Here's how the part is built. I have some questions about the finished solid (model axes, mm). Coordinates: 2 decimals unless noted, no trailing zeros. Order: outer loops, then holes, each group sorted by start corner. A loop starts at its lowest first (then second) coordinate and runs counter-clockwise, first axis right, second up. Notation, with made-up numbers: (29.5, 0.25) - (85.5, 0.25) arc R14 cw to (85.5, 6.25) - close; hole circle Ø10 at (2.5, 27). An arc over 180 degrees is marked (long way). Answer as CSV lines item,"result". Start each with the question number.
Q1. For pin 1 Ø1 at (y, z) = (-3, 29.5) entering from +X; pin 2 Ø1.5 at (x, z) = (-2.5, 28) entering from -Y, each with a flat end and sliding along its axis, tell me the tip position at first contact or that it passes through.
Q2. Suppose I cut it at B-B (z = 29.5). Please give me the cut outline in (x, y).
Q3. Thinking about a two-plate mould opening in Y: for faces 1 (the face through (6.466, -2.681, 28.779)), 2 (the face through (-1.3, 0.06, 28.14)), 3 (the face through (0, 0, 27.3)), which applies, released by +Y, released by -Y, zero draft, split by the parting line, or undercut?
Q4. I need wall thicknesses on line 1 (X direction, y = 2, z = 30.05); line 2 (X direction, y = -0.75, z = 28.3); line 3 (Y direction, x = 2.75, z = 27.7). Which ranges of each line are inside material? Lowest first, please.
Q5. Suppose I cut it at D-D (z = 27.85). Please give me the cut outline in (x, y).
Q6. Suppose I cut it at A-A (x = 2.75). Please give me the cut outline in (y, z).
Q7. Suppose I cut it at C-C (y = 0.5). Count the separate pieces of the cut face and the enclosed holes in it, then the cut area to 3 significant figures.
from build123d import *

# Parameters (mm, degrees)
SKETCH1_R                                            = 7
BOSS_EXTRUDE1_DEPTH                                  = 3
CSK_FOR_M2_5_COUNTERSUNK_FLAT_HEAD_SCREW_D           = 2.9
CSK_FOR_M2_5_COUNTERSUNK_FLAT_HEAD_SCREW_CSINK_D     = 5.5
CSK_FOR_M2_5_COUNTERSUNK_FLAT_HEAD_SCREW_CSINK_ANGLE = 90


with BuildPart() as part:
    # Sketch1 → Boss-Extrude1 (new body)
    with BuildSketch(Plane.XY.offset(27.3)):
        Circle(SKETCH1_R)
    extrude(amount=BOSS_EXTRUDE1_DEPTH)

    # CSK for M2.5 Countersunk Flat Head Screw1 (through all)
    with Locations(Plane.XY.offset(30.3)):
        with Locations((-2.75, 0), (2.75, 0)):
            CounterSinkHole(CSK_FOR_M2_5_COUNTERSUNK_FLAT_HEAD_SCREW_D / 2, CSK_FOR_M2_5_COUNTERSUNK_FLAT_HEAD_SCREW_CSINK_D / 2, counter_sink_angle=CSK_FOR_M2_5_COUNTERSUNK_FLAT_HEAD_SCREW_CSINK_ANGLE)


solid = part.part
Here are the results:
1,pin 1,"stops at x = 6.54"
1,pin 2,"stops at y = -6.78"
2,outline,"circle Ø14 at (0, 0); hole circle Ø3.9 at (-2.75, 0); hole circle Ø3.9 at (2.75, 0)"
3,face 1,"split by the parting line"
3,face 2,"undercut"
3,face 3,"zero draft"
4,line 1,"x = -6.71 to -4.25, -1.25 to 1.25, 4.25 to 6.71"
4,line 2,"x = -6.96 to -3.99, -1.51 to 1.51, 3.99 to 6.96"
4,line 3,"y = -6.44 to -1.45, 1.45 to 6.44"
5,outline,"circle Ø14 at (0, 0); hole circle Ø2.9 at (-2.75, 0); hole circle Ø2.9 at (2.75, 0)"
6,outline,"(-6.44, 27.3) - (-1.45, 27.3) - (-1.45, 29) - (-2.75, 30.3) - (-6.44, 30.3) - close; (1.45, 27.3) - (6.44, 27.3) - (6.44, 30.3) - (2.75, 30.3) - (1.45, 29) - close"
7,separate pieces,"3"
7,enclosed holes,"0"
7,area,"22.0 mm²"
